Build history of the part. All positions in model axes, mm. A direction names the side the tool comes from. Give positions to 0.01 mm unless a question says otherwise; leave off trailing zeros. Loops run counter-clockwise (first coordinate to the right, second up) from the corner with the lowest first, then second, coordinate; pieces in that order, holes last.
1) Wall check: line 1 (X direction, y = 1.4, z = -80); line 2 (Z direction, x = 11.5, y = 2.7); line 3 (X direction, y = 1.1, z = 50). Give the ranges that are in metal, low to high.
2) 3-axis set-ups, long thin cutter, end or side, ignore diameter. For faces 4 (the flat face through (135, 1, -65)), 5 (the flat face through (-64.67, 1.48, 47.37)): which of +Z, -Z, +X, -X, +Y, -Y reach the whole face in a straight line?
3) Flat gauge pins, fed straight in: P1, Ø2.5, axis at x = 67.66, z = 82.18, coming from the -Y side; P2, Ø6.5, axis at x = -51.01, z = 133.36, coming from the -Y side; P3, Ø1.5, axis at y = 2, z = 118.5, coming from the +X side; P4, Ø1.5, axis at y = 1.5, z = 97, coming from the -X side. Where does each tip first touch, or does it go through?
4) Two-plate mould, pull along Z, no slides. Class faces 1 (the flat face through (-108, 1, 137)), 2 (the flat face through (-64.423, 1.479, -49.226)), 3 (the flat face through (-135, 1, -65)): +Z half, -Z half, draft (parallel to the pull), parting line (faces both ways), or undercut.
5) Band-saw the part on A-A on z = 29. List the corners of the cut face in (x, y).
6) Band-saw the part on B-B on y = 2. State how many separate pieces and enclosed holes the cut face has, then the cut area to 3 significant figures.
```python
from build123d import *

# Parameters (mm, degrees)
BOSS_EXTRUDE1_DEPTH    = 3
SKETCH2_R              = 2.05
HEXCUT1_DEPTH          = 3
SKETCH5_R              = 1.55
CUT_EXTRUDE2_DEPTH     = 3
LPATTERN1_COUNT        = 2
LPATTERN1_PITCH        = 160
LPATTERN1_COUNT_DIR2   = 2
LPATTERN1_PITCH_DIR2   = 85
SKETCH6_R              = 2.05
QUADCUT1_DEPTH         = 3
SKETCH7_R              = 1.3
STDCARRIERCUBEFP_DEPTH = 3
CUT_EXTRUDE3_DEPTH     = 3
FILLET1_R              = 2
CIRPATTERN1_DEPTH      = 3
FILLET1_OF_MIRROR1_R   = 2


# Read off the part's stored shape, not the designer's step: CirPattern1
with BuildPart() as part:
    # Sketch1 → Boss-Extrude1 (new body)
    with BuildSketch(Plane(origin=(0, 0, 0), x_dir=(1, 0, 0), z_dir=(0, 1, 0))):
        Polygon((-95, 150), (-120, 125), (-120, 80), (-150, 50), (-150, -50), (-120, -80), (-120, -125), (-95, -150), (95, -150), (120, -125), (120, -80), (150, -50), (150, 50), (120, 80), (120, 125), (95, 150), align=None)
    extrude(amount=BOSS_EXTRUDE1_DEPTH)

    # Sketch2 → HexCut1 (cut)
    with BuildSketch(Plane(origin=(0, 3, 0), x_dir=(1, 0, 0), z_dir=(0, 1, 0))):
        with Locations(Location((51.014428415, 133.359581934, 0), (0, 0, 270))):
            Circle(SKETCH2_R)
        with Locations(Location((37.344555434, 99.682667397, 0), (0, 0, 270))):
            Circle(SKETCH2_R)
        with Locations(Location((37.344555434, -99.682667397, 0), (0, 0, 270))):
            Circle(SKETCH2_R)
        with Locations(Location((51.014428415, -133.359581934, 0), (0, 0, 270))):
            Circle(SKETCH2_R)
        with Locations(Location((105, 17.5, 0), (0, 0, 270))):
            Circle(SKETCH2_R)
        with Locations(Location((141, 22.5, 0), (0, 0, 270))):
            Circle(SKETCH2_R)
        with Locations(Location((105, -17.5, 0), (0, 0, 270))):
            Circle(SKETCH2_R)
        with Locations(Location((141, -22.5, 0), (0, 0, 270))):
            Circle(SKETCH2_R)
        with Locations(Location((89.985571585, -110.859581934, 0), (0, 0, 270))):
            Circle(SKETCH2_R)
        with Locations(Location((67.655444566, -82.182667397, 0), (0, 0, 270))):
            Circle(SKETCH2_R)
        with Locations(Location((89.985571585, 110.859581934, 0), (0, 0, 270))):
            Circle(SKETCH2_R)
        with Locations(Location((67.655444566, 82.182667397, 0), (0, 0, 270))):
            Circle(SKETCH2_R)
    hexcut1 = extrude(amount=-HEXCUT1_DEPTH, mode=Mode.SUBTRACT)

    # HexCut2: HexCut1 across plane
    add(hexcut1.mirror(Plane(origin=(0, 0, 0), x_dir=(0, 0, 1), z_dir=(1, 0, 0))), mode=Mode.SUBTRACT)

    # Sketch5 → Cut-Extrude2 (cut)
    with BuildSketch(Plane(origin=(0, 3, 0), x_dir=(1, 0, 0), z_dir=(0, 1, 0))):
        with Locations(Location((35, 80, 0), (0, 0, 270))):
            Circle(SKETCH5_R)
        with Locations(Location((50, 80, 0), (0, 0, 270))):
            Circle(SKETCH5_R)
    cut_extrude2 = extrude(amount=-CUT_EXTRUDE2_DEPTH, mode=Mode.SUBTRACT)

    # LPattern1: Cut-Extrude2 2 × 2
    with Locations(*[(-j * LPATTERN1_PITCH_DIR2, 0, i * LPATTERN1_PITCH) for i in range(LPATTERN1_COUNT) for j in range(LPATTERN1_COUNT_DIR2) if (i, j) != (0, 0)]):
        add(cut_extrude2, mode=Mode.SUBTRACT)

    # Sketch6 → QuadCut1 (cut)
    with BuildSketch(Plane(origin=(0, 3, 0), x_dir=(1, 0, 0), z_dir=(0, 1, 0))):
        with Locations(Location((86.620580695, 61.871843354, 0), (0, 0, 270))):
            Circle(SKETCH6_R)
        with Locations(Location((115.611958724, 83.792153571, 0), (0, 0, 270))):
            Circle(SKETCH6_R)
        with Locations(Location((83.792153571, 115.611958724, 0), (0, 0, 270))):
            Circle(SKETCH6_R)
        with Locations(Location((61.871843354, 86.620580695, 0), (0, 0, 270))):
            Circle(SKETCH6_R)
        with Locations(Location((86.620580695, -61.871843354, 0), (0, 0, 270))):
            Circle(SKETCH6_R)
        with Locations(Location((61.871843354, -86.620580695, 0), (0, 0, 270))):
            Circle(SKETCH6_R)
        with Locations(Location((83.792153571, -115.611958724, 0), (0, 0, 270))):
            Circle(SKETCH6_R)
        with Locations(Location((115.611958724, -83.792153571, 0), (0, 0, 270))):
            Circle(SKETCH6_R)
    quadcut1 = extrude(amount=-QUADCUT1_DEPTH, mode=Mode.SUBTRACT)

    # QuadCut2: QuadCut1 across plane
    add(quadcut1.mirror(Plane(origin=(0, 0, 0), x_dir=(0, 0, 1), z_dir=(1, 0, 0))), mode=Mode.SUBTRACT)

    # Sketch7 → StdCarrierCubeFP (cut)
    with BuildSketch(Plane(origin=(0, 3, 0), x_dir=(1, 0, 0), z_dir=(0, 1, 0))):
        with Locations(Location((-17.2, 42.5, 0), (0, 0, 270))):
            Circle(SKETCH7_R)
        with Locations(Location((17.2, 42.5, 0), (0, 0, 270))):
            Circle(SKETCH7_R)
        with Locations(Location((-17.2, -42.5, 0), (0, 0, 270))):
            Circle(SKETCH7_R)
        with Locations(Location((17.2, -42.5, 0), (0, 0, 270))):
            Circle(SKETCH7_R)
    extrude(amount=-STDCARRIERCUBEFP_DEPTH, mode=Mode.SUBTRACT)

    # Sketch8 → Cut-Extrude3 (cut)
    with BuildSketch(Plane(origin=(0, 3, 0), x_dir=(1, 0, 0), z_dir=(0, 1, 0))):
        Polygon((-17.5, -65), (17.5, -65), (22.5, -90), (-22.5, -90), align=None)
    cut_extrude3 = extrude(amount=-CUT_EXTRUDE3_DEPTH, mode=Mode.SUBTRACT)

    # Fillet1
    fillet1_edges = [part.edges().sort_by_distance(p)[0] for p in [
        (-22.5, 1.5, 90),
        (-17.5, 1.5, 65),
        (17.5, 1.5, 65),
        (22.5, 1.5, 90),
    ]]
    fillet(fillet1_edges, radius=FILLET1_R)

    # CirPattern1 outline → CirPattern1 (cut)
    with BuildSketch(Plane(origin=(0, 0, 0), x_dir=(1, 0, 0), z_dir=(0, 1, 0))):
        with BuildLine():
            ThreePointArc((54.915749171, -38.904044772), (54.849324183, -40.248979934), (55.650628912, -41.331187678))
            Line((55.650628912, -41.331187678), (73.444828679, -53.247833794))
            ThreePointArc((73.444828679, -53.247833794), (75.1372763, -53.500241806), (76.405467068, -52.351424618))
            Line((76.405467068, -52.351424618), (91.759026547, -15.284653092))
            ThreePointArc((91.759026547, -15.284653092), (91.67461668, -13.575570376), (90.299396073, -12.557308603))
            Line((90.299396073, -12.557308603), (69.290655474, -8.40125056))
            ThreePointArc((69.290655474, -8.40125056), (67.958811033, -8.599878987), (67.054767819, -9.59786132))
            Line((67.054767819, -9.59786132), (54.915749171, -38.904044772))
        make_face()
        with BuildLine():
            ThreePointArc((67.054767819, 11.617797575), (67.958811032, 10.619815242), (69.290655474, 10.421186816))
            Line((69.290655474, 10.421186816), (90.299396073, 14.577244859))
            ThreePointArc((90.299396073, 14.577244859), (91.67461668, 15.595506632), (91.759026547, 17.304589348))
            Line((91.759026547, 17.304589348), (76.405467068, 54.371360873))
            ThreePointArc((76.405467068, 54.371360873), (75.1372763, 55.520178061), (73.444828679, 55.267770049))
            Line((73.444828679, 55.267770049), (55.650628912, 43.351123933))
            ThreePointArc((55.650628912, 43.351123933), (54.849324183, 42.268916189), (54.915749171, 40.923981027))
            Line((54.915749171, 40.923981027), (67.054767819, 11.617797575))
        make_face()
        with BuildLine():
            ThreePointArc((-54.915749171, 40.923981027), (-54.849324183, 42.268916189), (-55.650628912, 43.351123933))
            Line((-55.650628912, 43.351123933), (-73.444828679, 55.267770049))
            ThreePointArc((-73.444828679, 55.267770049), (-75.1372763, 55.520178061), (-76.405467068, 54.371360873))
            Line((-76.405467068, 54.371360873), (-91.759026547, 17.304589348))
            ThreePointArc((-91.759026547, 17.304589348), (-91.67461668, 15.595506632), (-90.299396073, 14.577244859))
            Line((-90.299396073, 14.577244859), (-69.290655474, 10.421186816))
            ThreePointArc((-69.290655474, 10.421186816), (-67.958811032, 10.619815242), (-67.054767819, 11.617797575))
            Line((-67.054767819, 11.617797575), (-54.915749171, 40.923981027))
        make_face()
        with BuildLine():
            ThreePointArc((-67.054767819, -9.59786132), (-67.958811033, -8.599878987), (-69.290655474, -8.40125056))
            Line((-69.290655474, -8.40125056), (-90.299396073, -12.557308603))
            ThreePointArc((-90.299396073, -12.557308603), (-91.67461668, -13.575570376), (-91.759026547, -15.284653092))
            Line((-91.759026547, -15.284653092), (-76.405467068, -52.351424618))
            ThreePointArc((-76.405467068, -52.351424618), (-75.1372763, -53.500241806), (-73.444828679, -53.247833794))
            Line((-73.444828679, -53.247833794), (-55.650628912, -41.331187678))
            ThreePointArc((-55.650628912, -41.331187678), (-54.849324183, -40.248979934), (-54.915749171, -38.904044772))
            Line((-54.915749171, -38.904044772), (-67.054767819, -9.59786132))
        make_face()
    extrude(amount=CIRPATTERN1_DEPTH, mode=Mode.SUBTRACT)

    # Mirror1: Cut-Extrude3 across plane
    add(cut_extrude3.mirror(Plane.XY), mode=Mode.SUBTRACT)

    # Fillet1 of Mirror1
    fillet1_of_mirror1_edges = [part.edges().sort_by_distance(p)[0] for p in [
        (-22.5, 1.5, -90),
        (-17.5, 1.5, -65),
        (17.5, 1.5, -65),
        (22.5, 1.5, -90),
    ]]
    fillet(fillet1_of_mirror1_edges, radius=FILLET1_OF_MIRROR1_R)


solid = part.part
```
Findings below:
1. line 1: x = -120 to -51.55, -48.45 to -36.55, -33.45 to -20.5, 20.5 to 33.45, 36.55 to 48.45, 51.55 to 120
1. line 2: z = -150 to -90, -65 to 65, 90 to 150
1. line 3: x = -150 to -77.38, -68.6 to 68.6, 77.38 to 150
2. face 4: -Z, +X, +Y, -Y
2. face 5: +Y, -Y
3. P1: passes through
3. P2: stops at y = 0
3. P3: stops at x = 120
3. P4: stops at x = -120
4. face 1: +Z half
4. face 2: undercut
4. face 3: -Z half
5. outline: (-150, 0) - (-86.08, 0) - (-86.08, 3) - (-150, 3) - close; (-59.02, 0) - (59.02, 0) - (59.02, 3) - (-59.02, 3) - close; (86.08, 0) - (150, 0) - (150, 3) - (86.08, 3) - close
6. separate pieces: 1
6. enclosed holes: 58
6. area: 72,000 mm2
